The drawing under review shows one solid part. Ordinate dimensions are in mm from its lowest x, y, z. A direction names the side the tool comes from. Give positions to 0.01 mm unless a question says otherwise; leave off trailing zeros. Write each loop counter-clockwise with the first axis right and the second up, starting at its lowest first coordinate (ties: lowest second). Pieces come first, ordered by that corner, then holes. Notation, with made-up numbers: M 17,11.5 L 72,11.5 A13 cw 72,26.5 Z; hole C 69.25,88.25 d7. An arc over 180 degrees is marked long. Write item = value, one per line. Start each with the question number.
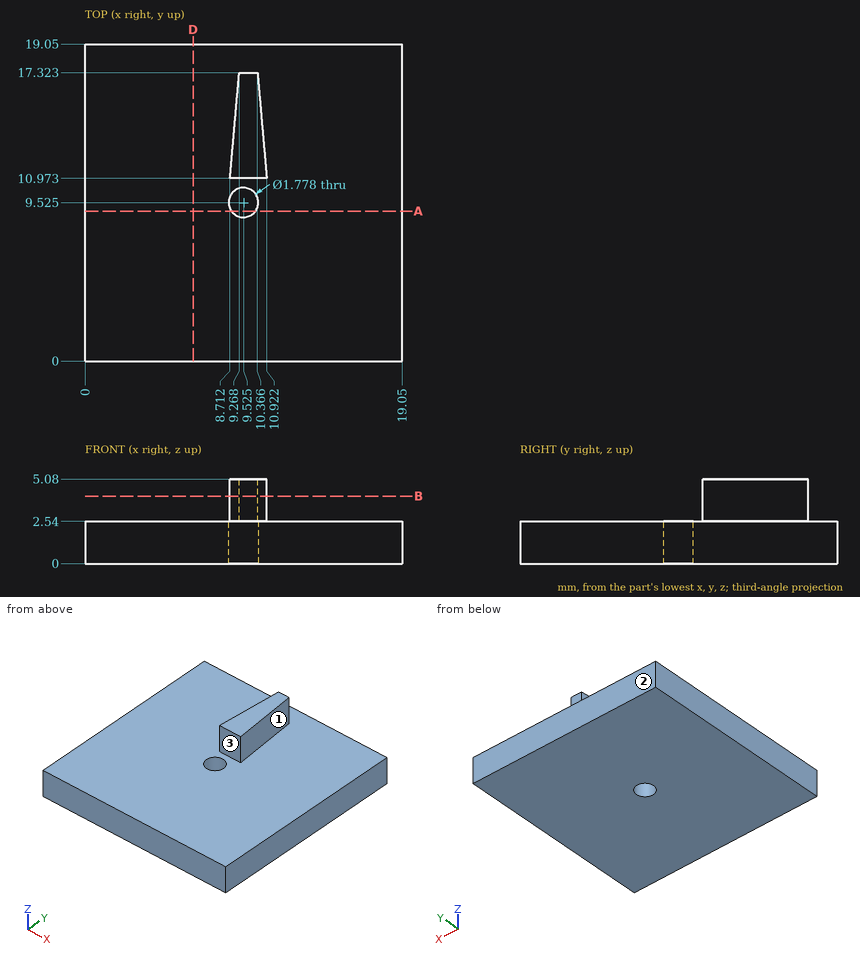
Item 1: Clearance check with flat-ended pins moving along their axes: P1, Ø1.1, axis at x = 9.525, y = 9.525, coming from the -Z side; P2, Ø0.7, axis at x = 10.5, z = 3.5, coming from the -Y side; P3, Ø3, axis at x = 3, y = 5, coming from the +Z side; P4, Ø1.2, axis at x = 10, z = 4, coming from the +Y side. State where each tip first meets the part, or that it passes through.
Item 2: For the marked faces 1, 2 and 3, list the 3-axis set-ups (+Z, -Z, +X, -X, +Y, -Y) from which the entire face can be reached by the end or side of a thin tool; tool diameter is ignored.
Item 3: We need section B-B, the plane z = 4.05. Write out the cut boundary in (x, y).
Item 4: We need section D-D, the plane x = 6.5. Write out the cut boundary in (y, z).
Item 5: To check wall thickness, follow probe 1 along Z at (x, y) = (14, 14); probe 2 along Y at (x, z) = (9, 0.9); probe 3 along X at (y, z) = (11.25, 3.8). State the ranges of each line that lie inside material, in increasing order. Write a range as [from, to].
Item 6: We need section A-A, the plane y = 9. Write out the cut boundary in (x, z).
Worked out:
q1.P1 = through
q1.P2 = 10.97
q1.P3 = 2.54
q1.P4 = 17.32
q2.face_1 = +Z, +X, +Y
q2.face_2 = +Z, -Z, +X, -X, +Y
q2.face_3 = +Z, +X, -X, -Y
q3.outline = M 8.71,10.97 L 10.92,10.97 L 10.37,17.32 L 9.27,17.32 Z
q4.outline = M 0,0 L 19.05,0 L 19.05,2.54 L 0,2.54 Z
q5.probe_1 = [0, 2.54]
q5.probe_2 = [0, 8.81], [10.24, 19.05]
q5.probe_3 = [8.74, 10.9]
q6.outline = M 0,0 L 8.81,0 L 8.81,2.54 L 0,2.54 Z; M 10.24,0 L 19.05,0 L 19.05,2.54 L 10.24,2.54 Z
